Design review of the part built by this model. Coordinates are the model's own, in mm. A direction names the side the tool comes from. Give positions to 0.01 mm unless a question says otherwise; leave off trailing zeros. Loops run counter-clockwise (first coordinate to the right, second up) from the corner with the lowest first, then second, coordinate; pieces in that order, holes last. Notation, with made-up numbers: (60, -14.5) - (64, -14.5) arc R18 ccw to (64, 2.5) - close; hole circle Ø9 at (2.25, -9). An arc over 180 degrees is marked (long way). Put each result on its own line as item: value. Start each with the question number.
```python
from build123d import *

# Parameters (mm, degrees)
BASE_FLANGE1_DEPTH           = 3.175
M8_CLEARANCE_HOLE1_D         = 9
EDGE_FLANGE1_DEPTH           = 16.378
EDGE_FLANGE2_STRIP_W         = 14.1732
EDGE_FLANGE2_STRIP_H         = 3.175
EDGE_FLANGE2_STRIP_CUT_DEPTH = 16.378
EDGE_FLANGE2_DEPTH           = 16.378
M5_CLEARANCE_HOLE1_D         = 5.5
FILLET1_R                    = 2.54


# Sheet-metal steps are written as plain solids
with BuildPart() as part:
    # Sketch1 → Base-Flange1 (new body)
    with BuildSketch(Plane.XY):
        Polygon((0, 0), (57.15, 0), (57.15, -16.378), (57.15, -29.184600001), (61.9125, -29.184600001), (61.9125, -45.562600001), (57.15, -45.562600001), (40.772, -45.562600001), (40.772, -16.378), (0, -16.378), align=None)
    extrude(amount=-BASE_FLANGE1_DEPTH)

    # M8 Clearance Hole1 (through all)
    with Locations(Plane.XY):
        with Locations((10, -8.189)):
            Hole(M8_CLEARANCE_HOLE1_D / 2)

    # Edge-Flange1 section (across the edge) → Edge-Flange1 (add)
    with BuildSketch(Plane(origin=(62.6491, -45.562600001, 0), x_dir=(-1, 0, 0), z_dir=(0, 1, 0))):
        with BuildLine():
            Line((-3.175, 0.7366), (-3.175, 23.9268))
            Line((-3.175, 23.9268), (0, 23.9268))
            Line((0, 23.9268), (0, 0.7366))
            ThreePointArc((0, 0.7366), (0.215745145, 0.215745145), (0.7366, 0))
            Line((0.7366, 0), (0.7366, -3.175))
            ThreePointArc((0.7366, -3.175), (-2.029318885, -2.029318885), (-3.175, 0.7366))
        make_face()
    extrude(amount=EDGE_FLANGE1_DEPTH)

    # Edge-Flange2 strip (across the edge) → Edge-Flange2 strip cut (cut)
    with BuildSketch(Plane(origin=(65.8241, -29.184600001, 23.9268), x_dir=(0, 0, -1), z_dir=(0, -1, 0))):
        with Locations((-6.35, -1.5875)):
            Rectangle(EDGE_FLANGE2_STRIP_W, EDGE_FLANGE2_STRIP_H)
    extrude(amount=EDGE_FLANGE2_STRIP_CUT_DEPTH, mode=Mode.SUBTRACT)

    # Edge-Flange2 section (across the edge) → Edge-Flange2 (add)
    with BuildSketch(Plane(origin=(65.8241, -29.184600001, 23.9268), x_dir=(0, 0, -1), z_dir=(0, -1, 0))):
        with BuildLine():
            Line((-3.175, 0.7366), (-3.175, 34.925))
            Line((-3.175, 34.925), (0, 34.925))
            Line((0, 34.925), (0, 0.7366))
            ThreePointArc((0, 0.7366), (0.215745145, 0.215745145), (0.7366, 0))
            Line((0.7366, 0), (0.7366, -3.175))
            ThreePointArc((0.7366, -3.175), (-2.029318885, -2.029318885), (-3.175, 0.7366))
        make_face()
    extrude(amount=EDGE_FLANGE2_DEPTH)

    # M5 Clearance Hole1 (through all)
    with Locations(Plane.XY.offset(27.1018)):
        with Locations((94.5499, -37.373600001)):
            Hole(M5_CLEARANCE_HOLE1_D / 2)

    # Fillet1
    fillet1_edges = [part.edges().sort_by_distance(p)[0] for p in [
        (0, 0, -1.5875),
        (57.15, 0, -1.5875),
        (57.15, -29.184600001, -1.5875),
        (40.772, -45.562600001, -1.5875),
        (40.772, -16.378, -1.5875),
        (0, -16.378, -1.5875),
        (100.7491, -29.184600001, 25.5143),
        (100.7491, -45.562600001, 25.5143),
    ]]
    fillet(fillet1_edges, radius=FILLET1_R)


solid = part.part
```
Item 1: Consider section B-B (z = 25.5). State the section outline as (x, y) points, plus the area to 3 significant figures.
Item 2: Machinability: for faces 4 (the flat face through (38, -12, 0)), 5 (the flat face through (40.772, -31, -2)), 6 (the flat face through (84, -37, 23.927)), which of the approach directions +Z, -Z, +X, -X, +Y, -Y give a long, thin tool a straight path to every point of the face, cutting with its end or side? Answer none if there is none.
Item 3: Consider section A-A (x = 10). State the section outline as (y, z) points (3 decimals), plus the area to 3 significant figures.
Item 4: For L1, parallel to Z at x = 68, y = -31; L2, parallel to X at y = -34, z = 1.5; L3, parallel to Z at x = 42.5, y = -7 (3 decimals), list the stretches that pass through material, from the lowest coordinate up. Write a range as from..to.
Item 5: Consider section D-D (y = -15). State the section outline as (x, z) points (3 decimals).
Item 6: Mouldability with a two-part tool opening along Y and no side actions: class faces 1 (the flat face through (83, -37, 27.102)), 2 (the cylindrical face through (0.764, -0.724, -1.61)), 3 (the cylindrical face through (97.3, -37.3, 25.5)) as pulls with the +Y half, pulls with the -Y half, needs draft (parallel to the pull), parting line crosses it, or undercut.
Item 7: For P1, Ø13, axis at y = -33.5, z = 9.5, coming from the +X side; P2, Ø12, axis at y = -18, z = 7, coming from the +X side; P3, Ø23, axis at x = 17.5, y = -19.5, coming from the +Z side; P4, Ø18, axis at x = 78.5, y = -41, coming from the -Z side, all flat-tipped, find the tip position at first contact; note any pin that passes through.
Item 8: Consider section C-C (z = 2). State the section outline as (x, y) points, plus the area to 3 significant figures.
Geometry says:
1. outline: (63.4, -45.56) - (98.21, -45.56) arc R2.54 ccw to (100.75, -43.02) - (100.75, -31.72) arc R2.54 ccw to (98.21, -29.18) - (63.4, -29.18) - close; hole circle Ø5.5 at (94.55, -37.37)
1. area: 585 mm2
2. face 4: +Z, -X, +Y, -Y
2. face 5: +Z, -Z, -X, -Y
2. face 6: -Z, +X, +Y, -Y
3. outline: (-16.378, -3.175) - (-12.689, -3.175) - (-12.689, 0) - (-16.378, 0) - close; (-3.689, -3.175) - (0, -3.175) - (0, 0) - (-3.689, 0) - close
3. area: 23.4 mm2
4. L1: z = 23.93..27.1
4. L2: x = 62.65..65.82
4. L3: z = -3.175..0
5. outline: (0.281, -3.175) - (57.15, -3.175) - (57.15, 0) - (0.281, 0) - close
6. face 1: needs draft
6. face 2: pulls with the +Y half
6. face 3: undercut
7. P1: stops at x = 65.82
7. P2: passes through
7. P3: stops at z = 0
7. P4: stops at z = 23.93
8. outline: (62.65, -45.56) - (65.82, -45.56) - (65.82, -29.18) - (62.65, -29.18) - close
8. area: 52.0 mm2
